Autodesk Inventor part; units mm, degrees
ref_plane "YZ Plane" through (0, 0, 0) normal (1, 0, 0) x (0, 1, 0)
ref_plane "XZ Plane" through (0, 0, 0) normal (0, 1, 0) x (-1, 0, 0)
ref_plane "XY Plane" through (0, 0, 0) normal (0, 0, 1) x (1, 0, 0)
sketch "スケッチ1" plane through (0, 0, 0) normal (0, 1, 0) x (-1, 0, 0)
  line L0 (8, 18) -> (-8, 18) construction
  line L1 (-8, 18) -> (-8, -18) construction
  line L2 (-8, -18) -> (8, -18) construction
  line L3 (8, -18) -> (8, 18) construction
  line L4 (8, 18) -> (-8, -18) construction
  line L5 (-8, 18) -> (8, -18) construction
  circle A0 centre (8, -18) radius 1.1
  circle A1 centre (-8, -18) radius 1.1
  circle A2 centre (8, 18) radius 1.1
  circle A3 centre (-8, 18) radius 1.1
  line L6 (13, 20) -> (-13, 20)
  line L7 (-13, 20) -> (-13, -20)
  line L8 (-13, -20) -> (13, -20)
  line L9 (13, -20) -> (13, 20)
  line L10 (13, 20) -> (-13, -20) construction
  line L11 (-13, 20) -> (13, -20) construction
  line L12 (8, -10) -> (-8, -10)
  line L13 (-8, -10) -> (-8, 15)
  line L14 (-8, 15) -> (8, 15)
  line L15 (8, 15) -> (8, -10)
  circle A4 centre (0, -10) radius 8
  point P0 (0, 0)
  dimension "d0" = 2.2
  dimension "d1" = 16
  dimension "d2" = 36
  dimension "d5" = 16
  dimension "d8" = 36
  dimension "d11" = 2
  dimension "d12" = 5
  dimension "d15" = 3
  dimension "d16" = 10
extrude "押し出し1" add sketch "スケッチ1" along normal blind 1.5
fillet "フィレット1" radius 2 2 edges at (8, 0.75, 15) (-8, 0.75, 15)
sketch "スケッチ2" plane through (0, 1.5, 0) normal (0, 1, 0) x (1, 0, 0)
  line L0 (-44, -7.75) -> (44, -7.75)
  line L1 (44, -7.75) -> (44, 30.75)
  line L2 (44, 30.75) -> (-44, 30.75)
  line L3 (-44, 30.75) -> (-44, -7.75)
  line L4 (-44, -7.75) -> (44, 30.75) construction
  line L5 (44, -7.75) -> (-44, 30.75) construction
  line L6 (13, 20) -> (-13, 20)
  line L7 (-13, 20) -> (-13, -20)
  line L8 (-8, -13) -> (-8, 10)
  line L9 (8, 10) -> (8, -13)
  line L10 (13, -20) -> (13, 20)
  line L11 (13, 20) -> (-13, 20)
  line L12 (-13, 20) -> (-13, -20)
  line L13 (-13, -20) -> (13, -20)
  circle A0 centre (-8, -18) radius 1.1
  circle A1 centre (8, -18) radius 1.1
  circle A2 centre (8, 18) radius 1.1
  circle A3 centre (-8, 18) radius 1.1
  line L14 (-8, -13) -> (-8, 10)
  arc A4 (8, 10) -> (-8, 10) centre (0, 10) ccw
  line L15 (8, 10) -> (8, -13)
  arc A5 (6, -15) -> (8, -13) centre (6, -13) ccw
  line L16 (6, -15) -> (-6, -15)
  arc A6 (-8, -13) -> (-6, -15) centre (-6, -13) ccw
  line L17 (33, 26.75) -> (23, 26.75)
  line L18 (23, 26.75) -> (23, 29.75)
  line L19 (23, 29.75) -> (33, 29.75)
  line L20 (33, 29.75) -> (33, 26.75)
  circle A7 centre (38, 28.25) radius 1.1
  line L21 (28, 26.75) -> (28, 29.75) construction
  circle A8 centre (18, 28.25) radius 1.1
  line L22 (44, 11.5) -> (-44, 11.5) construction
  line L23 (33, -3.75) -> (23, -3.75)
  line L24 (23, -3.75) -> (23, -6.75)
  line L25 (23, -6.75) -> (33, -6.75)
  line L26 (33, -6.75) -> (33, -3.75)
  circle A9 centre (38, -5.25) radius 1.1
  line L27 (28, -3.75) -> (28, -6.75) construction
  circle A10 centre (18, -5.25) radius 1.1
  line L28 (0, 30.75) -> (0, -7.75) construction
  line L29 (-33, 26.75) -> (-23, 26.75)
  line L30 (-23, 26.75) -> (-23, 29.75)
  line L31 (-23, 29.75) -> (-33, 29.75)
  line L32 (-33, 29.75) -> (-33, 26.75)
  circle A11 centre (-38, 28.25) radius 1.1
  line L33 (-28, 26.75) -> (-28, 29.75) construction
  circle A12 centre (-18, 28.25) radius 1.1
  circle A13 centre (-18, -5.25) radius 1.1
  line L34 (-23, -3.75) -> (-23, -6.75)
  line L35 (-28, -3.75) -> (-28, -6.75) construction
  line L36 (-33, -3.75) -> (-23, -3.75)
  line L37 (-23, -6.75) -> (-33, -6.75)
  line L38 (-33, -6.75) -> (-33, -3.75)
  circle A14 centre (-38, -5.25) radius 1.1
  circle A15 centre (-31.9, -6.75) radius 1.1
  circle A16 centre (-24.1, -6.75) radius 1.1
  line L39 (-33, -5.25) -> (-28, -5.25) construction
  circle A17 centre (-31.9, -3.75) radius 1.1
  circle A18 centre (-24.1, -3.75) radius 1.1
  circle A19 centre (-31.9, 29.75) radius 1.1
  circle A20 centre (-24.1, 29.75) radius 1.1
  circle A21 centre (-31.9, 26.75) radius 1.1
  circle A22 centre (-24.1, 26.75) radius 1.1
  circle A23 centre (31.9, -6.75) radius 1.1
  circle A24 centre (24.1, -6.75) radius 1.1
  circle A25 centre (31.9, -3.75) radius 1.1
  circle A26 centre (24.1, -3.75) radius 1.1
  circle A27 centre (31.9, 29.75) radius 1.1
  circle A28 centre (31.9, 26.75) radius 1.1
  circle A29 centre (24.1, 26.75) radius 1.1
  circle A30 centre (24.1, 29.75) radius 1.1
  line L40 (33, 29.75) -> (33, 30.75)
  line L41 (23, 29.75) -> (23, 30.75)
  line L42 (-33, 29.75) -> (-33, 30.75)
  line L43 (-23, 29.75) -> (-23, 30.75)
  line L44 (33, -6.75) -> (33, -7.75)
  line L45 (23, -6.75) -> (23, -7.75)
  line L46 (-33, -6.75) -> (-33, -7.75)
  line L47 (-23, -6.75) -> (-23, -7.75)
  point P0 (0, 0)
  point P1 (0, 11.5)
  point P2 (-13, -7.75)
  point P3 (13, -7.75)
  point P4 (33, 28.25)
  point P5 (33, -5.25)
  point P6 (-13, 20)
  point P7 (-13, 20)
  point P8 (-33, 28.25)
  point P9 (33, -3.75)
  point P10 (33, -6.75)
  point P11 (30.8, -6.75)
  point P12 (25.2, -6.75)
  point P13 (23, -6.75)
  point P14 (23, -3.75)
  point P15 (23, -3.75)
  point P16 (-23, 29.75)
  point P17 (-23, 26.75)
  point P18 (-25.2, 26.75)
  point P19 (-30.8, 26.75)
  point P20 (-33, 26.75)
  point P21 (-33, 29.75)
  point P22 (-23, -3.75)
  point P23 (-23, -6.75)
  point P24 (-25.2, -6.75)
  point P25 (-30.8, -6.75)
  point P26 (-33, -3.75)
  point P27 (33, 29.75)
  point P28 (33, 26.75)
  point P29 (30.8, 26.75)
  point P30 (25.2, 26.75)
  point P31 (23, 26.75)
  point P32 (23, 29.75)
  point P33 (23, 29.75)
  point P34 (24.2, -6.75)
  point P35 (-29.8, 26.75)
  point P36 (24.2, 26.75)
  point P37 (27.2, -3.75)
  point P38 (23, -6.75)
  point P39 (30.8, -3.75)
  point P40 (-25.2, 29.75)
  point P41 (-32.8, 29.75)
  point P42 (27.2, 29.75)
  point P43 (30.8, 29.75)
  point P44 (23, 26.75)
  point P45 (-32.8, -3.75)
  point P46 (26.2, -3.75)
  point P47 (-31.8, 29.75)
  point P48 (-31.8, -3.75)
  point P49 (-25.2, -3.75)
  point P50 (26.2, 29.75)
  point P51 (25.2, -3.75)
  point P52 (-30.8, 29.75)
  point P53 (-30.8, -3.75)
  point P54 (25.2, 29.75)
  point P55 (32.3583, 30.75)
  point P56 (23.6417, 30.75)
  point P57 (-23.6417, 30.75)
  point P58 (-32.3583, 30.75)
  point P59 (-32.3583, -7.75)
  point P60 (-23.6417, -7.75)
  point P61 (23.6417, -7.75)
  point P62 (32.3583, -7.75)
  dimension "d30" = 2.2
  dimension "d19" = 31
  dimension "d22" = 10
  dimension "d23" = 3
  dimension "d25" = 2.2
  dimension "d26" = 5
  dimension "d27" = 6
  dimension "d29" = 1
  dimension "d31" = 18.25
extrude "押し出し3" add sketch "スケッチ2" against normal blind 1.5 contours L3 L2 L42 L32 A21 L29 A22 L30 L43 L41 L18 A29 L17 A28 L20 L40 L1 L0 L44 L26 A25 L23 A26 L24 L45 L10 L6 L7 L47 L34 A18 L36 A17 L38 L46
fillet "フィレット2" radius 2 8 edges at (44, 0.75, -30.75) (44, 0.75, 7.75) (13, 0.75, 7.75) (13, 0.75, 20) (-13, 0.75, 20) (-13, 0.75, 7.75) (-44, 0.75, 7.75) (-44, 0.75, -30.75)
sketch "スケッチ4" plane through (0, 1.5, 0) normal (0, 1, 0) x (1, 0, 0)
  line L0 (41, 23.65) -> (11, 23.65)
  line L1 (11, 23.65) -> (11, -0.65)
  line L2 (11, -0.65) -> (41, -0.65)
  line L3 (41, -0.65) -> (41, 23.65)
  arc A0 (30.8, 26.75) -> (33, 26.75) centre (31.9, 26.75) ccw
  line L4 (44, -5.75) -> (44, 28.75)
  arc A1 (33, -3.75) -> (30.8, -3.75) centre (31.9, -3.75) ccw
  line L5 (-11, -20) -> (11, -20) construction
  line L6 (0, -20) -> (0, 21) construction
  line L7 (-41, 23.65) -> (-11, 23.65)
  line L8 (-11, 23.65) -> (-11, -0.65)
  line L9 (-11, -0.65) -> (-41, -0.65)
  line L10 (-41, -0.65) -> (-41, 23.65)
  line L11 (-44, -5.75) -> (-44, 28.75)
  line L12 (11, -0.65) -> (41, 23.65) construction
  line L13 (44, 24.7931) -> (12.5888, -0.65)
  line L14 (39.4112, 23.65) -> (11, 0.6369)
  line L15 (-44, 24.7931) -> (-12.5888, -0.65)
  line L16 (-39.4112, 23.65) -> (-11, 0.6369)
  line L17 (8, 10) -> (8, -13)
  point P0 (0, 0)
  point P1 (31.9, 25.65)
  point P2 (41, 11.5)
  point P3 (31.9, -2.65)
  point P4 (-41, 11.5)
  point P5 (-15, 23)
  point P6 (41, 22.3631)
  point P7 (39.7412, 23.9172)
  point P8 (11.3299, 0.9041)
  point P9 (-11.3299, 0.9041)
  point P10 (17, 0.7731)
  point P11 (-12.5888, -0.65)
  point P12 (-41, 22.3631)
  point P13 (-39.4112, 23.65)
  point P14 (-17, 0.7731)
  dimension "d39" = 2
  dimension "d40" = 3
  dimension "d41" = 2
  dimension "d43" = 1
  dimension "d48" = 3
extrude "押し出し5" cut sketch "スケッチ4" against normal blind 1.5 contours L14 L1 L0 | L3 L2 L13 | L7 L8 L16 | L15 L9 L10
fillet "フィレット3" radius 2 12 edges at (-39.4112, 0.75, -23.65) (-41, 0.75, -22.3631) (-11, 0.75, -23.65) (-12.5888, 0.75, 0.65) (-41, 0.75, 0.65) (41, 0.75, 0.65) (39.4112, 0.75, -23.65) (41, 0.75, -22.3631) (11, 0.75, -23.65) (12.5888, 0.75, 0.65) (-11, 0.75, -0.6369) (11, 0.75, -0.6369)
equation "\"d5\" = d1"
equation "\"d8\" = d2"
properties part number "KSHI" material "アルミニウム 2014-T4"
Source: CAD feature listing. Evaluate the final solid. Frame: model axes, mm. A direction names the side the tool comes from. Round coordinates to 2 decimals unless told otherwise and drop trailing zeros. Loops run counter-clockwise (first coordinate to the right, second up) from the corner with the lowest first, then second, coordinate; pieces in that order, holes last. Notation, with made-up numbers: (-31.75, -26) - (20.25, -26) arc R19 cw to (20.25, 10) - close; hole circle Ø5 at (81, 54). An arc over 180 degrees is marked (long way). Write item = value, one per line. Start each with the question number.
Item 1: Section query C-C on y = 0.6. Count the separate pieces of the cut face and the enclosed holes in it, plus the area to 3 significant figures.
Item 2: Mould query, pull axis Z, two halves, no side actions, for faces 1 (the face through (-43.43, 0.74, -30.15)), 2 (the face through (-7.43, 0.76, 14.4)), 3 (the face through (-43.4, 0.74, 7.18)), 4 (the face through (-39.89, 0.74, -19.96)). Classes: released by +Z, released by -Z, zero draft, split by the parting line, or undercut.
Item 3: First-contact query: pin 1 Ø12 at (x, z) = (20.5, -17.5) entering from +Y; pin 2 Ø0.8 at (x, y) = (-27.5, 0.5) entering from +Z. Flat tips, straight axial feed; report the tip coordinate or a pass-through.
Item 4: Section query B-B on x = 24.1. Output: boundary loops of the cut face in (y, z), plus the area to 3 significant figures.
Item 5: Material intervals for line 1 (X direction, y = 0.9, z = 0); line 2 (Z direction, x = 38, y = 0.4); line 3 (X direction, y = 0.55, z = -26.5), sorted ascending.
Item 6: Section query A-A on x = 0. Output: boundary loops of the cut face in (y, z), plus the area to 3 significant figures.
Item 7: Reachability of faces 5 (the face through (12.17, 0.74, -3.01)), 6 (the face through (12.4, 0.76, 19.43)) from +Z, -Z, +X, -X, +Y, -Y: full face, straight path, thin tool, end or side. Return the list, or none.
Results list:
q1.separate_pieces = 1
q1.enclosed_holes = 17
q1.area = 1,720 mm²
q2.face_1 = released by -Z
q2.face_2 = undercut
q2.face_3 = released by +Z
q2.face_4 = undercut
q3.pin_1 = through
q3.pin_2 = 3.75
q4.outline = (0, -25.65) - (1.5, -25.65) - (1.5, -23.65) - (0, -23.65) - close; (0, -11.25) - (1.5, -11.25) - (1.5, -8.67) - (0, -8.67) - close; (0, 0.65) - (1.5, 0.65) - (1.5, 2.65) - (0, 2.65) - close
q4.area = 9.86 mm²
q5.line_1 = -44 to -40.48, -16.76 to -8, 8 to 16.76, 40.48 to 44
q5.line_2 = -30.75 to -29.35, -27.15 to -19.9, 0.65 to 4.15, 6.35 to 7.75
q5.line_3 = -44 to -32.97, -30.83 to -25.17, -23.03 to 23.03, 25.17 to 30.83, 32.97 to 44
q6.outline = (0, -30.75) - (1.5, -30.75) - (1.5, -18) - (0, -18) - close; (0, 15) - (1.5, 15) - (1.5, 20) - (0, 20) - close
q6.area = 26.6 mm²
q7.face_5 = +Y, -Y
q7.face_6 = +Z, +X, +Y, -Y
